Could you check a few things on this model? Use its own coordinates, in mm. A direction names the side the tool comes from. Coordinates: 2 decimals unless noted, no trailing zeros. Order: outer loops, then holes, each group sorted by start corner. A loop starts at its lowest first (then second) coordinate and runs counter-clockwise, first axis right, second up. Notation, with made-up numbers: (60.5, -38.5) - (67.5, -38.5) arc R17 ccw to (67.5, -34.5) - close; hole circle Ø4 at (-34.5, 55.25). An arc over 180 degrees is marked (long way). Answer as a JSON object with one key per item and string values. Group by question number.
(1) Please list where these lines run through material, in increasing order: probe 1 along Z at (x, y) = (0.5, 1); probe 2 along Z at (x, y) = (-0.75, -1.75); probe 3 along X at (y, z) = (0, 3.5).
(2) Which directions (+Z, -Z, +X, -X, +Y, -Y) give clear straight access to the entire face, cutting with the end or side of a thin tool? Please do faces 1 (the flat face through (1.2, 1.2, -7.62)), 2 (the cylindrical face through (-0.19, -0.87, 7.73)), 3 (the cylindrical face through (-3.047, -0.134, -4.298)).
(3) Imagine slicing it at B-B, the plane z = 7.5. Write out the boundary of the cut face in (x, y).
(4) Imagine slicing it at A-A, the plane z = -8.5. Write out the boundary of the cut face in (x, y).
(5) Will this pin go through, and if not, where does the flat tip stop? P1, Ø1.5, axis at y = 1, z = 0.5, coming from the -X side.
Autodesk Inventor part; units mm, degrees
ref_plane "YZ Plane" through (0, 0, 0) normal (1, 0, 0) x (0, 1, 0)
ref_plane "XZ Plane" through (0, 0, 0) normal (0, 1, 0) x (-1, 0, 0)
ref_plane "XY Plane" through (0, 0, 0) normal (0, 0, 1) x (1, 0, 0)
sketch "Sketch1" plane through (0, 0, 0) normal (0, 1, 0) x (-1, 0, 0)
  line L0 (0, 0) -> (-3.05, 0)
  line L1 (-3.05, 0) -> (-3.05, -7.62)
  line L2 (-3.05, -7.62) -> (0, -7.62)
  line L3 (0, -7.62) -> (0, 0)
  line L4 (0, 0) -> (-0.889, 0)
  line L5 (-0.889, 0) -> (-0.889, 15.24)
  line L6 (-0.889, 15.24) -> (0, 15.24)
  line L7 (0, 15.24) -> (0, 0)
  line L8 (-0.889, 15.24) -> (0, 18.5578)
  line L9 (-0.889, 15.24) -> (2.5458, 15.24) construction
  line L10 (0, 18.5578) -> (0, 15.24)
  dimension "d0" = 3.05
  dimension "d1" = 7.62
  dimension "d2" = 0.889
  dimension "d3" = 15.24
  dimension "d13" = 75
  dimension "d14" = 15
  dimension "d15" = 18.5578
  dimension "d16" = 26.1778
revolve "Revolution1" add sketch "Sketch1" angle 360 about axis through (0, 0, 15.24) along (0, 0, -1)
sketch "Sketch2" plane through (0, 0, -7.62) normal (0, 0, -1) x (-1, 0, 0)
  circle A0 centre (0, 0) radius 3.05
  circle A1 centre (0, 0) radius 1.5
  dimension "d5" = 3
extrude "Extrusion1" add sketch "Sketch2" along normal blind 4 contours A1
chamfer "Chamfer1" distance 1.143 angle 45 1 edges at (-3.05, 0, 0)
chamfer "Chamfer2" distance 0.254 angle 45 1 edges at (-3.05, 0, -7.62)
thread "Thread1"
properties part number "carbide_probe_30deg_tip_r01" material "Steel, High Strength, Low Alloy"
Result set:
{
 "1": {"probe 1": "z = -11.62 to 0", "probe 2": "z = -7.62 to 0", "probe 3": "x = -0.89 to 0.89"},
 "2": {"face 1": "-Z", "face 2": "+Z", "face 3": "+Z, -Z"},
 "3": {"outline": "circle Ø1.78 at (0, 0)"},
 "4": {"outline": "circle Ø3 at (0, 0)"},
 "5": {"P1": "stops at x = -1.98"}
}
